from build123d import *

# Parameters (mm, degrees)
SKETCH1_W           = 44
SKETCH1_H           = 25
SKETCH1_W_2         = 40
SKETCH1_H_2         = 21
BOSS_EXTRUDE1_DEPTH = 26
BOSS_EXTRUDE2_DEPTH = 2
SKETCH3_W           = 17
SKETCH3_H           = 23
CUT_EXTRUDE1_DEPTH  = 57
SKETCH4_W           = 2.5
SKETCH4_H           = 1.8
BOSS_EXTRUDE3_DEPTH = 26
SKETCH8_W           = 25
SKETCH8_H           = 3
BOSS_EXTRUDE5_DEPTH = 15
SKETCH9_W           = 25
SKETCH9_H           = 3
BOSS_EXTRUDE6_DEPTH = 15


with BuildPart() as part:
    # Sketch1 → Boss-Extrude1 (new body)
    with BuildSketch(Plane(origin=(0, 0, 0), x_dir=(1, 0, 0), z_dir=(0, 1, 0))):
        with Locations((-20, 10.5)):
            Rectangle(SKETCH1_W, SKETCH1_H)
        with Locations((-20, 10.5)):
            Rectangle(SKETCH1_W_2, SKETCH1_H_2, mode=Mode.SUBTRACT)
    extrude(amount=BOSS_EXTRUDE1_DEPTH)

    # Sketch2 → Boss-Extrude2 (add)
    with BuildSketch(Plane.XY.offset(-21)):
        Polygon((-40, 22), (-36, 26), (-40, 26), align=None)
        Polygon((0, 26), (0, 22), (-4, 26), align=None)
    boss_extrude2 = extrude(amount=BOSS_EXTRUDE2_DEPTH)

    # Mirror1: Boss-Extrude2 across plane
    add(boss_extrude2.mirror(Plane(origin=(0, 0, -10.5), x_dir=(1, 0, 0), z_dir=(0, 0, -1))))

    # Sketch3 → Cut-Extrude1 (cut, symmetric)
    with BuildSketch(Plane(origin=(-40, 0, 0), x_dir=(0, 0, -1), z_dir=(1, 0, 0))):
        with Locations((10.5, 14.5)):
            Rectangle(SKETCH3_W, SKETCH3_H)
    extrude(amount=CUT_EXTRUDE1_DEPTH, both=True, mode=Mode.SUBTRACT)

    # Sketch4 → Boss-Extrude3 (add)
    with BuildSketch(Plane.XZ):
        with Locations((-24.25, -0.9)):
            Rectangle(SKETCH4_W, SKETCH4_H)
        with Locations((-15.75, -0.9)):
            Rectangle(SKETCH4_W, SKETCH4_H)
        with Locations((-15.75, -20.1)):
            Rectangle(SKETCH4_W, SKETCH4_H)
        with Locations((-24.25, -20.1)):
            Rectangle(SKETCH4_W, SKETCH4_H)
    extrude(amount=-BOSS_EXTRUDE3_DEPTH)

    # Sketch8 → Boss-Extrude5 (add)
    with BuildSketch(Plane(origin=(2, 0, 0), x_dir=(0, 0, -1), z_dir=(1, 0, 0))):
        with Locations((10.5, 1.5)):
            Rectangle(SKETCH8_W, SKETCH8_H)
    extrude(amount=BOSS_EXTRUDE5_DEPTH)

    # Sketch9 → Boss-Extrude6 (add)
    with BuildSketch(Plane.ZY.offset(42)):
        with Locations((-10.5, 1.5)):
            Rectangle(SKETCH9_W, SKETCH9_H)
    extrude(amount=BOSS_EXTRUDE6_DEPTH)


solid = part.part
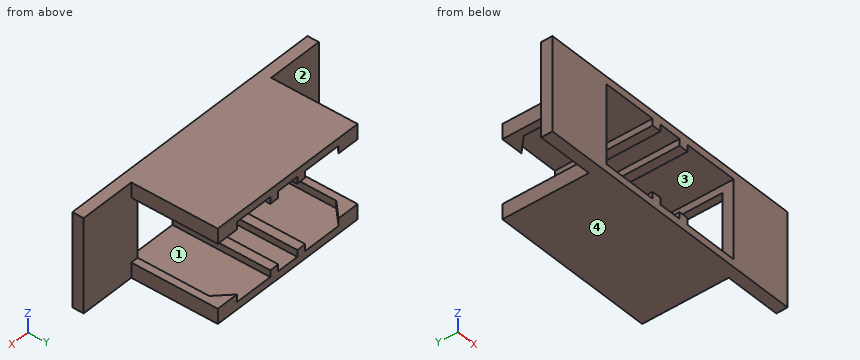
Read the model definition and answer for the solid it produces. Units are mm, in the model's axes. Face numbers are marked on the shaded views. A direction names the side the tool comes from. Give positions to 0.01 mm unless a question says otherwise; leave off trailing zeros. Loops run counter-clockwise (first coordinate to the right, second up) from the corner with the lowest first, then second, coordinate; pieces in that order, holes last. Notation, with made-up numbers: (-8, 86) - (51, 86) arc R13 cw to (51, 92) - close; hole circle Ø4 at (4.25, 8). An arc over 180 degrees is marked (long way). Answer as CSV lines item,"result". Start each with the question number.
1) Which of the six approach directions +Z, -Z, +X, -X, +Y, -Y give full straight-line access (tool end or side, diameter ignored) to the marked faces 3 and 4?
2) Each of these flat-tipped pins is pushed along its axis until it touches: pin 1 Ø2 at (y, z) = (7.5, -1) entering from +X; pin 2 Ø2 at (y, z) = (9.5, -0.5) entering from -X; pin 3 Ø4 at (x, z) = (-47.5, -13.5) entering from +Y; pin 4 Ø3 at (y, z) = (15.5, -17) entering from +X. Where does it stop, or does it pass through?
3) Determine the mould class of the marked faces 1 and 2 for opening direction X: released by +X, released by -X, zero draft, split by the parting line, or undercut.
4) Straight lines are drawn through the part: L1, parallel to X at y = 19.75, z = -20; L2, parallel to Z at x = -27.5, y = 18.25; L3, parallel to Z at x = -40.5, y = 16.5. For each, find the intervals that lie inside material, in ascending order. Write a range as from..to.
5) Find section C-C (z = -3.25). Write down the section's boundary in (x, y).
6) Find section A-A (x = -5). Write down the section's boundary in (y, z).
Findings below:
1,face 3,"-Y"
1,face 4,"-Z, +X, -X, +Y, -Y"
2,pin 1,"x = 2"
2,pin 2,"x = -42"
2,pin 3,"y = 3"
2,pin 4,"through"
3,face 1,"undercut"
3,face 2,"zero draft"
4,L1,"-42..-40, -25.5..-23, -17..-14.5, 0..2"
4,L2,"-23..-21, 0..2"
4,L3,"-23..-19, -2..2"
5,outline,"(-57, 0) - (-40, 0) - (-40, 3) - (-57, 3) - close; (0, 0) - (17, 0) - (17, 3) - (0, 3) - close"
6,outline,"(0, -23) - (26, -23) - (26, -21) - (0, -21) - close; (0, 0) - (26, 0) - (26, 2) - (0, 2) - close"
